The listing builds one solid part. Answer for the finished solid, in the listing's coordinates (mm). Face numbers are marked on the shaded views. A direction names the side the tool comes from. Round coordinates to 2 decimals unless told otherwise and drop trailing zeros. Write each loop counter-clockwise with the first axis right and the second up, starting at its lowest first coordinate (ties: lowest second). Pieces come first, ordered by that corner, then holes. Notation, with made-up numbers: (-27, 60.25) - (6, 60.25) arc R14 cw to (6, 66.25) - close; hole circle Ø6 at (49, 76.5). An arc over 180 degrees is marked (long way). Use a Markdown table: item, result. Add a question column.
1) Find the intervals of material crossed by probe 1 along X at (y, z) = (60.5, 1114.5); probe 2 along Z at (x, y) = (-751.5, -98); probe 3 along Y at (x, z) = (659, 1311), in increasing order. Write a range as from..to.
2) A cutting plane is placed at C-C (x = -37). Give the vertices of the cut face in (y, z).
3) Determine the mould class of the marked faces 1, 2 and 3 for opening direction X: +X half, -X half, draft (parallel to the pull), parting line (faces both ways), or undercut.
4) Each of these flat-tipped pins is pushed along its axis until it touches: P1, Ø4, axis at x = -276, y = 67, coming from the +Z side; P2, Ø12, axis at x = 108.5, z = 1486.5, coming from the -Y side. Where does it stop, or does it pass through?
5) A cutting plane is placed at A-A (y = 255). Give the vertices of the cut face in (x, z), then the cut area to 3 significant figures.
6) A cutting plane is placed at B-B (z = 1627.5). Give the vertices of the cut face in (x, y), then the cut area to 3 significant figures.
7) A tool of negligible diameter and unlimited length cuts with its end or side. For the marked faces 4 and 5, from which of +Z, -Z, +X, -X, +Y, -Y can it reach the whole face along a straight path? Write none if from no direction.
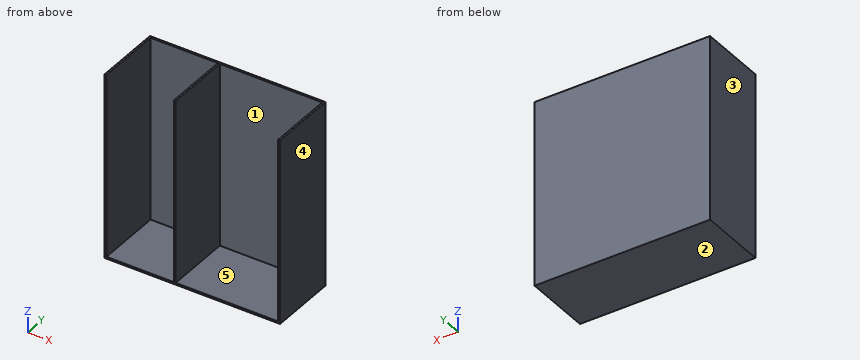
```python
from build123d import *

# Parameters (mm, degrees)
F0_W     = 647.7
F0_H     = 635
F1_DEPTH = 18.034
F0_W_2   = 985.266
F0_W_3   = 18.034
F2_DEPTH = 1778


with BuildPart() as f1:
    # F0 (on Top) → F1 (new body)
    with BuildSketch(Plane.XY):
        with Locations((-501.65, 0)):
            Rectangle(F0_W, F0_H)
    extrude(amount=F1_DEPTH)



with BuildPart() as f1b:
    # F0 (on Top) → F1, piece 2 (new body)
    with BuildSketch(Plane.XY):
        with Locations((332.867, 0)):
            Rectangle(F0_W_2, F0_H)
    extrude(amount=F1_DEPTH)


with BuildPart() as f1_1:
    add(f1.part)

    add(f1b.part)  # F2 merges F1b
    # F0 (on Top) → F2 (join)
    with BuildSketch(Plane.XY):
        with Locations((-834.517, 0)):
            Rectangle(F0_W_3, F0_H)
        with Locations((834.517, 0)):
            Rectangle(F0_W_3, F0_H)
        Polygon((-843.534, 317.5), (-825.5, 317.5), (-177.8, 317.5), (-159.766, 317.5), (825.5, 317.5), (843.534, 317.5), (843.534, 335.534), (-843.534, 335.534), align=None)
        with Locations((-168.783, 0)):
            Rectangle(F0_W_3, F0_H)
    extrude(amount=F2_DEPTH)


solid = f1_1.part
```
Entries:
| question | item | result |
|---|---|---|
| 1 | probe 1 | x = -843.53..-825.5, -177.8..-159.77, 825.5..843.53 |
| 1 | probe 2 | z = 0..18.03 |
| 1 | probe 3 | y = 317.5..335.53 |
| 2 | outline | (-317.5, 0) - (335.53, 0) - (335.53, 1778) - (317.5, 1778) - (317.5, 18.03) - (-317.5, 18.03) - close |
| 3 | face 1 | undercut |
| 3 | face 2 | draft |
| 3 | face 3 | -X half |
| 4 | P1 | stops at z = 18.03 |
| 4 | P2 | stops at y = 317.5 |
| 5 | outline | (-843.53, 0) - (843.53, 0) - (843.53, 1778) - (825.5, 1778) - (825.5, 18.03) - (-159.77, 18.03) - (-159.77, 1778) - (-177.8, 1778) - (-177.8, 18.03) - (-825.5, 18.03) - (-825.5, 1778) - (-843.53, 1778) - close |
| 5 | area | 126,000 mm² |
| 6 | outline | (-843.53, -317.5) - (-825.5, -317.5) - (-825.5, 317.5) - (-177.8, 317.5) - (-177.8, -317.5) - (-159.77, -317.5) - (-159.77, 317.5) - (825.5, 317.5) - (825.5, -317.5) - (843.53, -317.5) - (843.53, 335.53) - (-843.53, 335.53) - close |
| 6 | area | 64,800 mm² |
| 7 | face 4 | +Z, -Z, +X, +Y, -Y |
| 7 | face 5 | +Z, -Y |
